```python
from build123d import *

# Parameters (mm, degrees)
SKETCH_1_R          = 2.5
EXTRUDE_1_DEPTH     = 2
EXTRUDE_2_DEPTH     = 30
SKETCH_4_R          = 6
CUT_EXTRUDE_1_DEPTH = 15


with BuildPart() as part:
    # 草图1 → 凸台-拉伸1 (new body)
    with BuildSketch(Plane.XY):
        Polygon((-30.821938658, 18.493163195), (-0.821938658, 18.493163195), (-0.821938658, 8.493163195), (-0.821938658, -1.506836805), (-30.821938658, -1.506836805), align=None)
        with Locations((-25.821938658, 8.493163195)):
            Circle(SKETCH_1_R, mode=Mode.SUBTRACT)
        with Locations((-5.821938658, 8.493163195)):
            Circle(SKETCH_1_R, mode=Mode.SUBTRACT)
    extrude(amount=EXTRUDE_1_DEPTH)

    # 草图2 → 凸台-拉伸2 (add)
    with BuildSketch(Plane.XY.offset(2)):
        Polygon((-22.821938658, 3.493163195), (-8.821938658, 3.493163195), (-8.821938658, 13.493163195), (-15.821938658, 13.493163195), (-22.821938658, 13.493163195), align=None)
    extrude(amount=EXTRUDE_2_DEPTH)

    # 草图4 → 切除-拉伸1 (cut)
    with BuildSketch(Plane.XZ.offset(-3.493163195)):
        with Locations((-15.821938658, 22)):
            Circle(SKETCH_4_R)
    extrude(amount=-CUT_EXTRUDE_1_DEPTH, mode=Mode.SUBTRACT)


solid = part.part
```
The model under review builds one solid part; all positions refer to its coordinate system, in mm. A direction names the side the tool comes from. Round coordinates to 2 decimals unless told otherwise and drop trailing zeros. Loops run counter-clockwise (first coordinate to the right, second up) from the corner with the lowest first, then second, coordinate; pieces in that order, holes last. Notation, with made-up numbers: M 23,46.5 L 45,46.5 A30 cw 45,78.5 Z; hole C 57.25,47 d8. An arc over 180 degrees is marked long. Put each result on its own line as item: value.
Q1. Consider section A-A, the plane z = 22. Give the boundary of the cut face in (x, y).
Result set:
outline: M -22.82,3.49 L -21.82,3.49 L -21.82,13.49 L -22.82,13.49 Z; M -9.82,3.49 L -8.82,3.49 L -8.82,13.49 L -9.82,13.49 Z
Q2. Consider section D-D, the plane z = 7. Give the boundary of the cut face in (x, y), then the cut area to 3 significant figures.
Result set:
outline: M -22.82,3.49 L -8.82,3.49 L -8.82,13.49 L -22.82,13.49 Z
area: 140 mm²
Q3. Mouldability with a two-part tool opening along X and no side actions: class faces 1 (the flat face through (-8.822, 8, 17)), 2 (the flat face through (-16, 2, 2)), 3 (the cylindrical face through (-10.28, 8.42, 19.7)), 4 (the flat face through (-22.822, 9, 17)) as released by +X, released by -X, zero draft, split by the parting line, or undercut.
Result set:
face 1: released by +X
face 2: zero draft
face 3: undercut
face 4: released by -X
Q4. Consider section B-B, the plane y = 6.5. Give the boundary of the cut face in (x, z).
Result set:
outline: M -30.82,0 L -27.33,0 L -27.33,2 L -30.82,2 Z; M -24.31,0 L -7.33,0 L -7.33,2 L -8.82,2 L -8.82,32 L -22.82,32 L -22.82,2 L -24.31,2 Z; M -4.31,0 L -0.82,0 L -0.82,2 L -4.31,2 Z; hole C -15.82,22 d12
Q5. Consider section C-C, the plane x = -16.5. Give the boundary of the cut face in (y, z), then the cut area to 3 significant figures.
Result set:
outline: M -1.51,0 L 18.49,0 L 18.49,2 L 13.49,2 L 13.49,16.04 L 3.49,16.04 L 3.49,2 L -1.51,2 Z; M 3.49,27.96 L 13.49,27.96 L 13.49,32 L 3.49,32 Z
area: 221 mm²
Q6. Machinability: for faces 5 (the flat face through (-30.822, 8, 1)), 6 (the flat face through (-16, 13.493, 13)), 7 (the flat face through (-16, 3.493, 13)), which of the approach directions +Z, -Z, +X, -X, +Y, -Y give a long, thin tool a straight path to every point of the face, cutting with its end or side? Answer none if there is none.
Result set:
face 5: +Z, -Z, -X, +Y, -Y
face 6: +Z, +X, -X, +Y
face 7: +Z, +X, -X, -Y
Q7. To check wall thickness, follow L1, parallel to Z at x = -16, y = 11.5; L2, parallel to Z at x = -3.75, y = 5.75; L3, parallel to Y at x = -9.75, z = 12. State the ranges of each line that lie inside material, in increasing order.
Result set:
L1: z = 0 to 16, 28 to 32
L2: z = 0 to 2
L3: y = 3.49 to 13.49
Q8. For pin 1 (11 mm diameter, centred on y = 7.5, z = 19.5, fed in from +X); pin 2 (15.5 mm diameter, centred on x = -14.5, z = 21, fed in from -Y); pin 3 (15.5 mm diameter, centred on x = -15.82, z = 22, fed in from +Y), all flat-tipped, find the tip position at first contact; note any pin that passes through.
Result set:
pin 1: stops at x = -8.82
pin 2: stops at y = 3.49
pin 3: stops at y = 13.49
